CAD build for the part. Positions are in the model's coordinates, mm. Face numbers are marked on the shaded views. A direction names the side the tool comes from. Give positions to 0.01 mm unless a question says otherwise; leave off trailing zeros. Order: outer loops, then holes, each group sorted by start corner. A loop starts at its lowest first (then second) coordinate and runs counter-clockwise, first axis right, second up. Notation, with made-up numbers: M 34.5,-5.75 L 68.5,-5.75 A25 ccw 68.5,10.25 Z; hole C 49,58.5 d2. An arc over 180 degrees is marked long. Put each result on its own line as item: value. Start each with the question number.
1) Drill centre lines: line 1 (Z direction, x = 3.1, y = -15); line 2 (Y direction, x = 4.45, z = -4); line 3 (Y direction, x = 3, z = 3.5). Where is each one in solid material? Low to high. Write a range as [from, to].
2) Cut at D-D (x = 14). Write the cut outline in (y, z), and give its area (3 significant figures).
3) Tool access for the marked faces 1, 2, 3, 4 and 5: list every direction of +Z, -Z, +X, -X, +Y, -Y with a clear straight run to the whole face (end or side of a thin tool).
4) Two-plate mould, pull along Z, no slides. Class the marked faces 6, 7, 8 and 9: released by +Z, released by -Z, zero draft, split by the parting line, or undercut.
5) Cut at A-A (y = -9.75). Write the cut outline in (x, z).
6) Pin check, flat tips, straight feed: pin 1 (2.5 mm diameter, centred on y = -3.5, z = -2, fed in from +X); pin 2 (5 mm diameter, centred on x = 20, y = -0.5, fed in from +Z); pin 3 (4 mm diameter, centred on x = 12, z = 20, fed in from +Y); pin 4 (2.5 mm diameter, centred on y = -15, z = 44, fed in from +X). Stop position of each tip, or through.
7) Cut at B-B (z = 44). Write the cut outline in (x, y).
8) Cut at C-C (y = -5). Write the cut outline in (x, z), and give its area (3 significant figures).
Autodesk Inventor part; units mm, degrees
ref_plane "YZ Plane" through (0, 0, 0) normal (1, 0, 0) x (0, 1, 0)
ref_plane "XZ Plane" through (0, 0, 0) normal (0, 1, 0) x (-1, 0, 0)
ref_plane "XY Plane" through (0, 0, 0) normal (0, 0, 1) x (1, 0, 0)
sketch "Sketch1" plane through (0, 0, 0) normal (1, 0, 0) x (0, 1, 0)
  line L0 (0, 0) -> (0, 40)
  line L1 (0, 40) -> (-20, 40)
  line L2 (-20, 40) -> (-20, 43)
  line L3 (-15, 48) -> (-2, 48)
  line L4 (-2, -8) -> (-15, -8)
  line L5 (-20, -3) -> (-20, 0)
  line L6 (-20, 0) -> (0, 0)
  line L7 (0, 20) -> (3, 20)
  line L8 (3, 20) -> (3, 25.5)
  line L9 (3, 23.7768) -> (3, 20)
  line L10 (3, 20) -> (3, 16.2232)
  line L11 (3, 20) -> (7.9, 20)
  line L12 (7.9, 20) -> (7.9, 22.7)
  line L13 (7.9, 22.7) -> (7.9, 20)
  line L14 (7.9, 20) -> (7.9, 17.3)
  line L15 (7.9, 20) -> (10.6, 20) construction
  line L16 (4.4961, 24.6451) -> (7.9, 22.7)
  line L17 (7.9, 17.3) -> (4.4961, 15.3549)
  line L18 (7.9, 17.3) -> (7.9, 12.3)
  line L19 (7.9, 12.3) -> (5.5193, 10.9396)
  line L20 (7.9, 22.7) -> (7.9, 27.7)
  line L21 (7.9, 27.7) -> (5.5193, 29.0604)
  line L22 (3, 43) -> (3, 33.4016)
  line L23 (3, 30.5) -> (3, 25.5)
  line L24 (3, 14.5) -> (3, 9.5)
  line L25 (3, 6.5984) -> (3, -3)
  arc A0 (3, 33.4016) -> (5.5193, 29.0604) centre (8, 33.4016) ccw
  arc A1 (5.5193, 10.9396) -> (3, 6.5984) centre (8, 6.5984) ccw
  arc A2 (-2, -8) -> (3, -3) centre (-2, -3) ccw
  arc A3 (3, 43) -> (-2, 48) centre (-2, 43) ccw
  arc A4 (-15, 48) -> (-20, 43) centre (-15, 43) ccw
  arc A5 (-20, -3) -> (-15, -8) centre (-15, -3) ccw
  arc A6 (3, 16.2232) -> (4.4961, 15.3549) centre (4, 16.2232) ccw
  arc A7 (4.4961, 24.6451) -> (3, 23.7768) centre (4, 23.7768) ccw
  point P0 (-20, 48)
  point P1 (3, 48)
  point P2 (3, -8)
  point P3 (-20, -8)
  point P4 (-20, -1.5)
  dimension "d0" = 40
  dimension "d1" = 20
  dimension "d2" = 8
  dimension "d3" = 23
  dimension "d5" = 56
  dimension "d6" = 23
  dimension "d7" = 5.5
  dimension "d8" = 5.5
  dimension "d9" = 4.9
  dimension "d10" = 2.7
  dimension "d11" = 2.7
  dimension "d13" = 5
  dimension "d14" = 5
  dimension "d15" = 17.5
  dimension "d16" = 17.5
  dimension "d17" = 5
  dimension "d18" = 5
  dimension "d19" = 5
  dimension "d20" = 5
  dimension "d45" = 1
extrude "Extrusion1" add sketch "Sketch1" along normal blind 23 contours L0 L7 L10 A6 L17 L18 L19 A1 L25 A2 L4 A5 L5 L6 | L0 L1 L2 A4 L3 A3 L22 A0 L21 L20 L16 A7 L8 L7
sketch "Sketch2" plane through (0, 0, 0) normal (0, -1, 0) x (1, 0, 0)
  line L0 (0, 48) -> (23, 48)
  line L1 (0, 48) -> (6, 48)
  line L2 (6, 48) -> (6, -8)
  line L3 (0, -8) -> (23, -8)
  line L4 (0, 6.5984) -> (23, 6.5984)
  line L5 (23, 34.6451) -> (23, 6.5984)
  line L6 (23, 6.5984) -> (6, 0)
  line L7 (0, 0) -> (23, 0)
  line L8 (23, 33.4016) -> (23, 43)
  line L9 (23, 33.4016) -> (6, 40)
  line L10 (0, 40) -> (23, 40)
  line L11 (6, 48) -> (23, 48)
  line L12 (23, 33.4016) -> (23, 29.0604)
  line L13 (23, 33.4016) -> (23, 48)
  line L14 (23, 6.5984) -> (23, -8)
  line L15 (23, 40) -> (23, 0)
  line L16 (6, -8) -> (23, -8)
  dimension "d23" = 6
extrude "Extrusion2" cut sketch "Sketch2" along normal blind 23 and the other way blind 11.5 contours L0 L13 L8 L10 L2 | L10 L8 L5 L9 | L7 L14 L3 L2 | L6 L14 L7
fillet "Fillet1" radius 5 4 edges at (23, 1.5, 6.5984) (23, 1.5, 33.4016) (6, 1.5, 40) (6, 1.5, 0)
sketch "Sketch3" plane through (0, 0, 0) normal (-1, 0, 0) x (0, 0, 1)
  line L0 (40, 0) -> (0, 0)
  line L1 (40, 0) -> (40, -5)
  line L2 (40, -20) -> (40, 0)
  line L3 (40, -5) -> (44, -5)
  line L4 (44, -5) -> (44, -15)
  line L5 (0, 0) -> (0, -5)
  line L6 (0, 0) -> (0, -20)
  line L7 (0, -5) -> (-4, -5)
  line L8 (-4, -5) -> (-4, -15)
  dimension "d29" = 5
  dimension "d30" = 4
  dimension "d31" = 10
  dimension "d32" = 5
  dimension "d33" = 4
  dimension "d34" = 10
hole "Hole1" at (0, -15, 44) at (0, -5, 44) at (0, -15, -4) at (0, -5, -4) direction (1, 0, 0) diameter 4 depth 15
sketch "Sketch4" plane through (6, -15, -8) normal (1, 0, 0) x (0, 0, -1)
  line L0 (-0.0094, 15) -> (-56.0094, 15)
  line L1 (-56.0094, 15) -> (-56.0094, -8.2095)
  line L2 (-56.0094, -8.2095) -> (-0.0094, -8.2095)
  line L3 (-0.0094, -8.2095) -> (-0.0094, 15)
  point P0 (-8, 15)
  dimension "d42" = 56
extrude "Extrusion3" cut sketch "Sketch4" along normal blind 23
properties part number "bigServoHolder2"
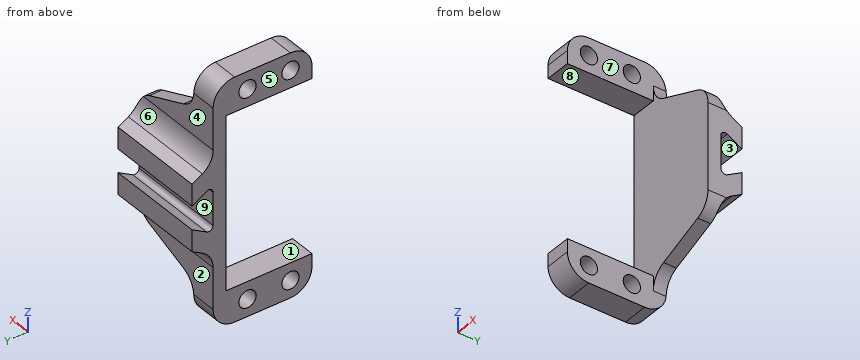
Solution:
1. line 1: [-8, -6], [-2, 0], [40, 42], [46, 48]
1. line 2: [-19.9, -17], [-13, -7], [-3, 2.9]
1. line 3: [0, 3]
2. outline: M 0,3.11 L 3,3.11 L 3,6.6 A5 cw 5.52,10.94 L 7.9,12.3 L 7.9,17.3 L 4.5,15.35 A1 cw 3,16.22 L 3,23.78 A1 cw 4.5,24.65 L 7.9,22.7 L 7.9,27.7 L 5.52,29.06 A5 cw 3,33.4 L 3,36.89 L 0,36.89 Z
2. area: 154 mm²
3. face 1: +X, -X, -Y
3. face 2: -Z, +X, -X, +Y
3. face 3: +X, -X
3. face 4: +Z, +X, -X, +Y
3. face 5: +Z, -Z, -X, +Y, -Y
4. face 6: released by +Z
4. face 7: zero draft
4. face 8: undercut
4. face 9: undercut
5. outline: M 0,-8 L 6,-8 L 6,0 L 0,0 Z; M 0,40 L 6,40 L 6,48 L 0,48 Z
6. pin 1: x = 6
6. pin 2: z = 35.52
6. pin 3: y = 3
6. pin 4: through
7. outline: M 0,-19.9 L 6,-19.9 L 6,-17 L 0,-17 Z; M 0,-13 L 6,-13 L 6,-7 L 0,-7 Z; M 0,-3 L 6,-3 L 6,2.9 L 0,2.9 Z
8. outline: M 0,-8 L 6,-8 L 6,-6 L 0,-6 Z; M 0,-2 L 6,-2 L 6,0 L 0,0 Z; M 0,40 L 6,40 L 6,42 L 0,42 Z; M 0,46 L 6,46 L 6,48 L 0,48 Z
8. area: 48.0 mm²
